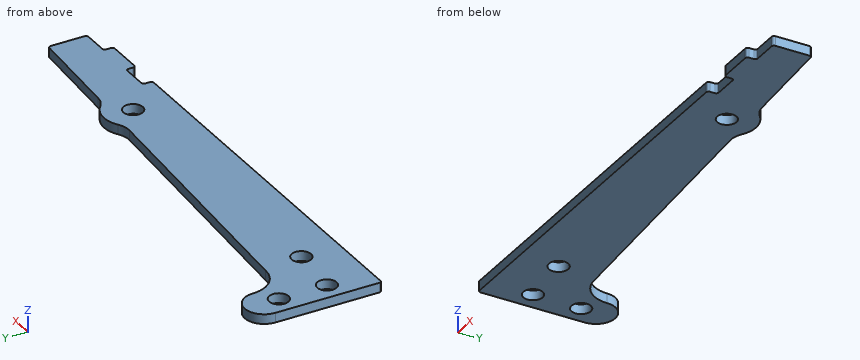
```python
from build123d import *

# Parameters (mm, degrees)
SKETCH1_R           = 1.5875
BOSS_EXTRUDE1_DEPTH = 1.5875
FILLET1_R           = 0.4064
FILLET2_R           = 3.571875


with BuildPart() as part:
    # Sketch1 → Boss-Extrude1 (new body)
    with BuildSketch(Plane.XY):
        with BuildLine():
            Line((0, -1.5875), (65.4074384, -1.5875))
            Line((65.4074384, -1.5875), (65.4074384, 0))
            Line((65.4074384, 0), (70.1699384, 0))
            Line((70.1699384, 0), (70.1699384, -1.5875))
            Line((70.1699384, -1.5875), (76.5199384, -1.5875))
            Line((76.5199384, -1.5875), (76.5199384, 0))
            Line((76.5199384, 0), (81.2824384, 0))
            Line((81.2824384, 0), (81.2824384, 6.35))
            Line((81.2824384, 6.35), (63.718396184, 7.542088136))
            ThreePointArc((63.718396184, 7.542088136), (60.17368185, 9.514068607), (56.395022028, 8.039132457))
            Line((56.395022028, 8.039132457), (11.1125, 11.1125))
            ThreePointArc((11.1125, 11.1125), (7.744903955, 12.507403955), (6.35, 15.875))
            ThreePointArc((6.35, 15.875), (3.175, 19.05), (0, 15.875))
            Line((0, 15.875), (0, -1.5875))
        make_face()
        with Locations((3.175, 5.588)):
            Circle(SKETCH1_R, mode=Mode.SUBTRACT)
        with Locations((3.175, 13.462)):
            Circle(SKETCH1_R, mode=Mode.SUBTRACT)
        with Locations((11.90625, 4.7625)):
            Circle(SKETCH1_R, mode=Mode.SUBTRACT)
        with Locations((59.8511884, 4.7625)):
            Circle(SKETCH1_R, mode=Mode.SUBTRACT)
    extrude(amount=BOSS_EXTRUDE1_DEPTH)

    # Fillet1
    fillet1_edges = [part.edges().sort_by_distance(p)[0] for p in [
        (81.2824384, 6.35, 0.79375),
        (81.2824384, 0, 0.79375),
        (76.5199384, 0, 0.79375),
        (76.5199384, -1.5875, 0.79375),
        (70.1699384, -1.5875, 0.79375),
        (70.1699384, 0, 0.79375),
        (65.4074384, 0, 0.79375),
        (65.4074384, -1.5875, 0.79375),
        (0, -1.5875, 0.79375),
    ]]
    fillet(fillet1_edges, radius=FILLET1_R)

    # Fillet2
    fillet2_edges = [part.edges().sort_by_distance(p)[0] for p in [
        (56.395022028, 8.039132457, 0.79375),
        (63.718396184, 7.542088136, 0.79375),
    ]]
    fillet(fillet2_edges, radius=FILLET2_R)


solid = part.part
```
Input: part model. Units: mm. Frame: model coordinates. Give positions to 0.01 mm unless a question says otherwise; leave off trailing zeros. Write each loop counter-clockwise with the first axis right and the second up, starting at its lowest first coordinate (ties: lowest second). Pieces come first, ordered by that corner, then holes. Notation, with made-up numbers: (29.25, -24) - (50.25, -24) arc R18 cw to (50.25, -6) - close; hole circle Ø9 at (89, -10). An arc over 180 degrees is marked (long way). Write item = value, one per line. Start each with the question number.
1. Section query B-B, the plane x = 17. Output: boundary loops of the cut face in (y, z).
2. Ray query, L1, parallel to Y at x = 23, z = 0.9; L2, parallel to Y at x = 34.5, z = 1; L3, parallel to X at y = 11.75, z = 0.95. Return the intervals inside material, ascending.
3. First-contact query: pin 1 Ø1.9 at (x, y) = (3.175, 5.588) entering from -Z; pin 2 Ø0.9 at (y, z) = (-1, 1) entering from +X; pin 3 Ø0.8 at (x, z) = (78.5, 0.5) entering from -Y. Flat tips, straight axial feed; report the tip coordinate or a pass-through.
4. Section query C-C, the plane x = 28. Output: boundary loops of the cut face in (y, z), then the cut area to 3 significant figures.
5. Section query A-A, the plane z = 0.3. Count the separate pieces of the cut face and the enclosed holes in it, then the cut area to 3 significant figures.
Check sheet entries:
q1.outline = (-1.59, 0) - (10.71, 0) - (10.71, 1.59) - (-1.59, 1.59) - close
q2.L1 = -1.59 to 10.31
q2.L2 = -1.59 to 9.53
q2.L3 = 0 to 8.73
q3.pin_1 = through
q3.pin_2 = 76.52
q3.pin_3 = 0
q4.outline = (-1.59, 0) - (9.97, 0) - (9.97, 1.59) - (-1.59, 1.59) - close
q4.area = 18.3 mm2
q5.separate_pieces = 1
q5.enclosed_holes = 4
q5.area = 878 mm2
